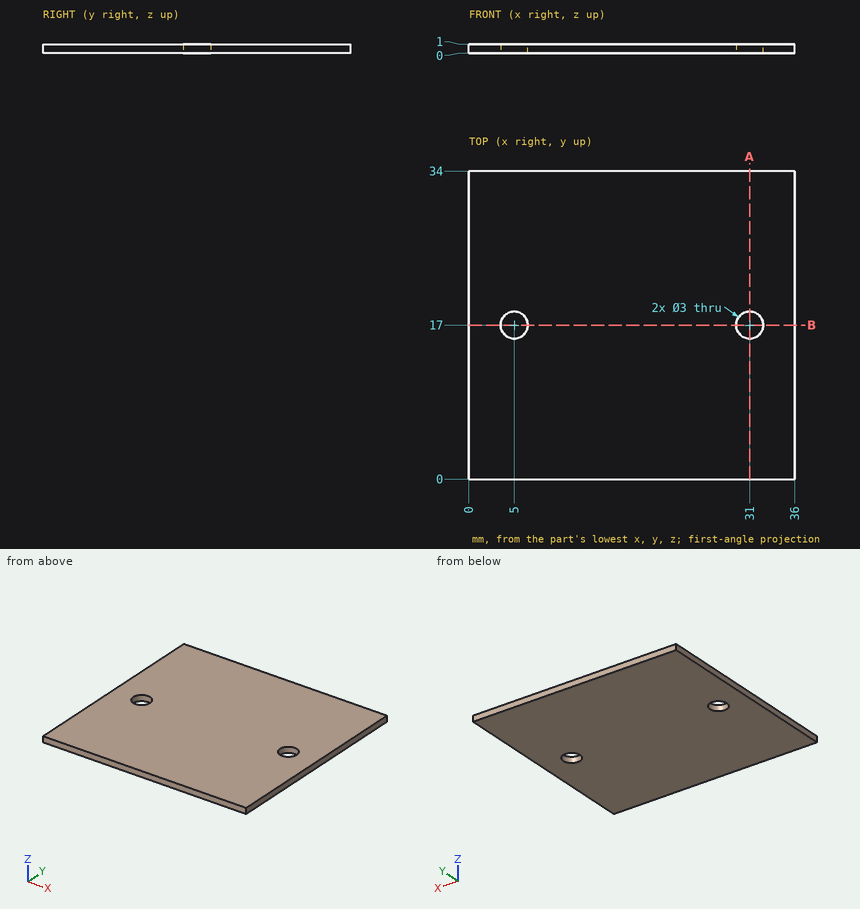
Drawing for the job (mm, zero at the part's lowest x, y, z). Round coordinates to 2 decimals unless told otherwise and drop trailing zeros. Write each loop counter-clockwise with the first axis right and the second up, starting at its lowest first coordinate (ties: lowest second). Pieces come first, ordered by that corner, then holes. Notation, with made-up numbers: (33.5, 37.25) - (72.5, 37.25) arc R26 cw to (72.5, 66.25) - close; hole circle Ø10 at (85, -10.5). An arc over 180 degrees is marked (long way). Use CSV: the item, a comma, the result in double quotes.
(1) Band-saw the part on A-A (x = 31). Write the cut outline in (y, z), plus the area to 3 significant figures.
Response:
outline,"(0, 0) - (15.5, 0) - (15.5, 1) - (0, 1) - close; (18.5, 0) - (34, 0) - (34, 1) - (18.5, 1) - close"
area,"31.0 mm²"
(2) Wall check: line 1 (X direction, y = 17, z = 0.75); line 2 (Y direction, x = 5, z = 0.25); line 3 (X direction, y = 17.5, z = 0.9). Give the ranges that are in metal, low to high.
Response:
line 1,"0 to 3.5, 6.5 to 29.5, 32.5 to 36"
line 2,"0 to 15.5, 18.5 to 34"
line 3,"0 to 3.59, 6.41 to 29.59, 32.41 to 36"
(3) Pin check, flat tip, straight feed: P1, Ø2.5, axis at x = 31, y = 17, coming from the -Z side. Stop position of the tip, or through.
Response:
P1,"through"
(4) Band-saw the part on B-B (y = 17). Write the cut outline in (x, z), plus the area to 3 significant figures.
Response:
outline,"(0, 0) - (3.5, 0) - (3.5, 1) - (0, 1) - close; (6.5, 0) - (29.5, 0) - (29.5, 1) - (6.5, 1) - close; (32.5, 0) - (36, 0) - (36, 1) - (32.5, 1) - close"
area,"30.0 mm²"
